Model file for the job. Use its own axes, mm. A direction names the side the tool comes from. Round coordinates to 2 decimals unless told otherwise and drop trailing zeros. Order: outer loops, then holes, each group sorted by start corner. A loop starts at its lowest first (then second) coordinate and runs counter-clockwise, first axis right, second up. Notation, with made-up numbers: (19.25, 16) - (60.25, 16) arc R15 ccw to (60.25, 38) - close; hole circle Ø1 at (-0.75, 17.25). An arc over 180 degrees is marked (long way). Answer as CSV lines item,"result". Start each with the question number.
1. Band-saw the part on A-A on z = -2. List the corners of the cut face in (x, y).
2. 3-axis set-ups, long thin cutter, end or side, ignore diameter. For faces 5 (the face through (-68, 2, 18.75)), 6 (the face through (80, 2, -7.5)), 7 (the face through (25.5, 2, -21)), 8 (the face through (24, 2, 18.75)): which of +Z, -Z, +X, -X, +Y, -Y reach the whole face in a straight line?
3. Band-saw the part on C-C on x = 29.5. List the corners of the cut face in (y, z).
4. Pin check, flat tips, straight feed: pin 1 Ø1.2 at (y, z) = (2, -23.5) entering from +X; pin 2 Ø2 at (y, z) = (1.5, 20) entering from -X; pin 3 Ø2 at (y, z) = (2.5, 21) entering from +X. Stop position of each tip, or through.
5. Pull direction X, two halves, no side cores. Call faces 1 (the face through (-83, 2, 9)), 2 (the face through (-25.5, 2, 21)), 3 (the face through (-38, 2, -18.75)), 4 (the face through (20, 2, 23.75)): released by +X, released by -X, zero draft, split by the parting line, or undercut.
6. Wall check: line 1 along X through (y, z) = (2, -19); line 2 along X through (y, z) = (2.3, 19); line 3 along Z through (x, y) = (72.5, 3.75). Give the ranges that are in metal, low to high. Write a range as [from, to].
7. Band-saw the part on B-B on y = 3.25. State how many separate pieces and enclosed holes the cut face has, then the cut area to 3 significant figures.
```python
from build123d import *

# Parameters (mm, degrees)
SKETCH1_W           = 24.5
SKETCH1_H           = 4
BOSS_EXTRUDE1_DEPTH = 4
FILLET1_R           = 1


with BuildPart() as part:
    # Sketch1 → Boss-Extrude1 (new body)
    with BuildSketch(Plane(origin=(0, 0, 0), x_dir=(1, 0, 0), z_dir=(0, 1, 0))):
        Polygon((-53, 18.75), (-78, 18.75), (-78, 11.5), (-83, 11.5), (-83, 7.5), (-78, 7.5), (-78, 4.5), (-83, 4.5), (-83, -4.5), (-78, -4.5), (-78, -7.5), (-83, -7.5), (-83, -11.5), (-78, -11.5), (-78, -18.75), (-57, -18.75), (-57, -23.75), (-53, -23.75), (-53, -18.75), (-50, -18.75), (-50, -23.75), (-25.5, -23.75), (-25.5, -18.75), (-22.5, -18.75), (-22.5, -23.75), (-18.5, -23.75), (-18.5, -18.75), (18.5, -18.75), (18.5, -23.75), (22.5, -23.75), (22.5, -18.75), (25.5, -18.75), (25.5, -23.75), (50, -23.75), (50, -18.75), (53, -18.75), (53, -23.75), (57, -23.75), (57, -18.75), (78, -18.75), (78, -11.5), (83, -11.5), (83, -7.5), (78, -7.5), (78, -4.5), (83, -4.5), (83, 4.5), (78, 4.5), (78, 7.5), (83, 7.5), (83, 11.5), (78, 11.5), (78, 18.75), (53, 18.75), (53, 25.75), (22.5, 25.75), (22.5, 18.75), (-22.5, 18.75), (-22.5, 25.75), (-53, 25.75), align=None)
        with Locations((37.75, 20.75)):
            Rectangle(SKETCH1_W, SKETCH1_H, mode=Mode.SUBTRACT)
        with Locations((-37.75, 20.75)):
            Rectangle(SKETCH1_W, SKETCH1_H, mode=Mode.SUBTRACT)
        Polygon((-12.935798956, 14.75), (-74, -14.607788964), (-74, 14.75), align=None, mode=Mode.SUBTRACT)
        Polygon((-3, 15.088558194), (-3, -14.75), (-65.064201044, -14.75), align=None, mode=Mode.SUBTRACT)
        Polygon((3, -14.75), (3, 15.088558194), (65.064201044, -14.75), align=None, mode=Mode.SUBTRACT)
        Polygon((74, -14.607788964), (12.935798956, 14.75), (74, 14.75), align=None, mode=Mode.SUBTRACT)
    extrude(amount=BOSS_EXTRUDE1_DEPTH)

    # Fillet1
    fillet1_edges = [part.edges().sort_by_distance(p)[0] for p in [
        (-74, 2, 14.607788964),
        (-12.935798956, 2, -14.75),
        (-74, 2, -14.75),
        (65.064201044, 2, 14.75),
        (3, 2, -15.088558194),
        (3, 2, 14.75),
        (12.935798956, 2, -14.75),
        (74, 2, 14.607788964),
        (74, 2, -14.75),
        (-65.064201044, 2, 14.75),
        (-3, 2, 14.75),
        (-3, 2, -15.088558194),
    ]]
    fillet(fillet1_edges, radius=FILLET1_R)


solid = part.part
```
Reply:
1,outline,"(-83, 0) - (-74, 0) - (-74, 4) - (-83, 4) - close; (-39.46, 0) - (-30.22, 0) - (-30.22, 4) - (-39.46, 4) - close; (-3, 0) - (3, 0) - (3, 4) - (-3, 4) - close; (30.22, 0) - (39.46, 0) - (39.46, 4) - (30.22, 4) - close; (74, 0) - (83, 0) - (83, 4) - (74, 4) - close"
2,face 5,"+Z, -X, +Y, -Y"
2,face 6,"+X, +Y, -Y"
2,face 7,"+Y, -Y"
2,face 8,"+Z, +Y, -Y"
3,outline,"(0, -25.75) - (4, -25.75) - (4, -22.75) - (0, -22.75) - close; (0, -18.75) - (4, -18.75) - (4, -14.75) - (0, -14.75) - close; (0, -6.79) - (4, -6.79) - (4, -2.35) - (0, -2.35) - close; (0, 14.75) - (4, 14.75) - (4, 23.75) - (0, 23.75) - close"
4,pin 1,"stops at x = 53"
4,pin 2,"stops at x = -57"
4,pin 3,"stops at x = 57"
5,face 1,"released by -X"
5,face 2,"undercut"
5,face 3,"undercut"
5,face 4,"zero draft"
6,line 1,"x = [-53, -50], [-25.5, -22.5], [22.5, 25.5], [50, 53]"
6,line 2,"x = [-57, -53], [-50, -25.5], [-22.5, -18.5], [18.5, 22.5], [25.5, 50], [53, 57]"
6,line 3,"z = [-18.75, -14.75], [13.89, 18.75]"
7,separate pieces,"1"
7,enclosed holes,"6"
7,area,"2,950 mm2"
